from build123d import *

# Parameters (mm, degrees)
BOSS_EXTRUDE1_DEPTH = 30
FILLET2_R           = 2
SKETCH3_R           = 1.5
CUT_EXTRUDE4_DEPTH  = 9
SKETCH4_R           = 1.35
CUT_EXTRUDE3_DEPTH  = 33
FILLET3_R           = 1


with BuildPart() as part:
    # Sketch1 → Boss-Extrude1 (new body)
    with BuildSketch(Plane(origin=(0, 0, 0), x_dir=(1, 0, 0), z_dir=(0, 1, 0))):
        Polygon((-21.5, 0.5), (8.5, 0.5), (8.5, 7.5), (9.5, 7.5), (9.5, 0.5), (9.5, -0.5), (-22.5, -0.5), (-22.5, 0.5), (-22.5, 7.5), (-21.5, 7.5), align=None)
    extrude(amount=BOSS_EXTRUDE1_DEPTH)

    # Fillet2
    fillet2_edges = [part.edges().sort_by_distance(p)[0] for p in [
        (9.5, 15, 0.5),
        (-22.5, 15, 0.5),
        (-21.5, 15, -0.5),
        (8.5, 15, -0.5),
    ]]
    fillet(fillet2_edges, radius=FILLET2_R)

    # Sketch3 → Cut-Extrude4 (cut, through all)
    with BuildSketch(Plane.XY.offset(0.5)):
        with Locations((-14, 25)):
            Circle(SKETCH3_R)
        with Locations((1, 25)):
            Circle(SKETCH3_R)
        with Locations((-14, 5)):
            Circle(SKETCH3_R)
        with Locations((1, 5)):
            Circle(SKETCH3_R)
    extrude(amount=-CUT_EXTRUDE4_DEPTH, mode=Mode.SUBTRACT)

    # Sketch4 → Cut-Extrude3 (cut, through all)
    with BuildSketch(Plane(origin=(9.5, 0, 0), x_dir=(0, 0, -1), z_dir=(1, 0, 0))):
        with Locations((4.5, 26)):
            Circle(SKETCH4_R)
        with Locations((4.5, 4)):
            Circle(SKETCH4_R)
    extrude(amount=-CUT_EXTRUDE3_DEPTH, mode=Mode.SUBTRACT)

    # Fillet3
    fillet3_edges = [part.edges().sort_by_distance(p)[0] for p in [
        (9, 30, -7.5),
        (-22, 0, -7.5),
        (9, 0, -7.5),
        (-22, 30, -7.5),
    ]]
    fillet(fillet3_edges, radius=FILLET3_R)


solid = part.part
Model file for the job. Use its own axes, mm. A direction names the side the tool comes from. Coordinates: 2 decimals unless noted, no trailing zeros. Order: outer loops, then holes, each group sorted by start corner. A loop starts at its lowest first (then second) coordinate and runs counter-clockwise, first axis right, second up. Notation, with made-up numbers: (2, 16) -> (39, 16) arc R8 ccw to (39, 24) -> close; hole circle Ø10 at (72, 11). An arc over 180 degrees is marked (long way). Return JSON: item names as keys, results as strings. Group by question number.
Item 1: Flat gauge pin, fed straight in: P1, Ø8, axis at x = -7.5, y = 15, coming from the -Z side. Where does the tip first touch, or does it go through?
Item 2: Saw through at D-D on y = 2. Write the cut outline in (x, z).
Item 3: Wall check: line 1 along Y through (x, z) = (-14, 0.3); line 2 along Y through (x, z) = (-21.9, -4.5); line 3 along X through (y, z) = (7.75, -2.75). Give the ranges that are in metal, low to high. Write a range as [from, to].
Item 4: Saw through at C-C on z = -1. Write the cut outline in (x, y), then the cut area to 3 significant figures.
Item 5: Saw through at A-A on y = 24. Write the cut outline in (x, z).
Item 6: Saw through at B-B on x = 1. Write the cut outline in (y, z).
Item 7: Pull direction Y, two halves, no side cores. Call faces 1 (the cylindrical face through (-21.99, 2.8, -5.12)), 2 (the flat face through (-6, 30, 0)), 3 (the flat face through (-22.5, 15, -5)): pulls with the +Y half, pulls with the -Y half, needs draft (parallel to the pull), parting line crosses it, or undercut.
Item 8: Tool access for faces 4 (the cylindrical face through (0.805, 26.487, 0.007)), 5 (the cylindrical face through (-20.9, 15.21, -1.07)): list every direction of +Z, -Z, +X, -X, +Y, -Y with a clear straight run to the whole face (end or side of a thin tool).
Values found:
{
 "1": {"P1": "stops at z = -0.5"},
 "2": {"outline": "(-22.5, -7.5) -> (-21.5, -7.5) -> (-21.5, -2.5) arc R2 cw to (-19.5, -0.5) -> (6.5, -0.5) arc R2 cw to (8.5, -2.5) -> (8.5, -7.5) -> (9.5, -7.5) -> (9.5, -1.5) arc R2 ccw to (7.5, 0.5) -> (-20.5, 0.5) arc R2 ccw to (-22.5, -1.5) -> close"},
 "3": {"line 1": "y = [0, 3.5], [6.5, 23.5], [26.5, 30]", "line 2": "y = [0, 2.65], [5.35, 24.65], [27.35, 30]", "line 3": "x = [-22.5, -21.5], [8.5, 9.5]"},
 "4": {"outline": "(-22.44, 0) -> (-20.82, 0) -> (-20.82, 30) -> (-22.44, 30) -> close; (7.82, 0) -> (9.44, 0) -> (9.44, 30) -> (7.82, 30) -> close", "area": "96.8 mm2"},
 "5": {"outline": "(-22.5, -7.5) -> (-21.5, -7.5) -> (-21.5, -2.5) arc R2 cw to (-19.5, -0.5) -> (-15.12, -0.5) -> (-15.12, 0.5) -> (-20.5, 0.5) arc R2 ccw to (-22.5, -1.5) -> close; (-12.88, -0.5) -> (-0.12, -0.5) -> (-0.12, 0.5) -> (-12.88, 0.5) -> close; (2.12, -0.5) -> (6.5, -0.5) arc R2 cw to (8.5, -2.5) -> (8.5, -7.5) -> (9.5, -7.5) -> (9.5, -1.5) arc R2 ccw to (7.5, 0.5) -> (2.12, 0.5) -> close"},
 "6": {"outline": "(0, -0.5) -> (3.5, -0.5) -> (3.5, 0.5) -> (0, 0.5) -> close; (6.5, -0.5) -> (23.5, -0.5) -> (23.5, 0.5) -> (6.5, 0.5) -> close; (26.5, -0.5) -> (30, -0.5) -> (30, 0.5) -> (26.5, 0.5) -> close"},
 "7": {"face 1": "undercut", "face 2": "pulls with the +Y half", "face 3": "needs draft"},
 "8": {"face 4": "+Z, -Z", "face 5": "-Z, +Y, -Y"}
}
